Could you check a few things on this model? Use its own coordinates, in mm. Give positions to 0.01 mm unless a question says otherwise; leave off trailing zeros. Order: outer loops, then holes, each group sorted by start corner. A loop starts at its lowest first (then second) coordinate and runs counter-clockwise, first axis right, second up. Notation, with made-up numbers: M 56.25,66.25 L 110.25,66.25 A24 ccw 110.25,98.25 Z; hole C 52.5,12.25 d1. An arc over 180 degrees is marked long. Use a Markdown table: item, result. Add a question column.
Item 1: If I drill on L1, parallel to Y at x = 4.75, z = -1.5; L2, parallel to X at y = -14, z = 4.5; L3, parallel to Y at x = 6.5, z = -1.25, over which ranges is the centre line in solid material (lowest first)? Write a range as from..to.
Item 2: I'm going to push flat-ended pins straight in: pin 1 Ø0.6 at (x, y) = (1, -99) entering from +Z; pin 2 Ø2 at (y, z) = (-168, -12) entering from -X; pin 3 Ø1.5 at (x, y) = (4, -85.5) entering from +Z. Where does each tip first touch, or does it pass through?
Item 3: If we mould it in two halves opening along Z, with no side actions, what happens to faces 1 (the face through (4.056, -249.768, -3.294)), 2 (the face through (5, -271.216, -2)), 3 (the face through (4.056, -242.268, -3.294))? For each: released by +Z, released by -Z, zero draft, split by the parting line, or undercut.
Item 4: Suppose I cut it at B-B on x = 3.5. Write out the boundary of the cut face in (y, z).
Item 5: Suppose I cut it at A-A on y = -134.5. Write out the boundary of the cut face in (x, z), plus the area to 3 significant figures.
from build123d import *

# Parameters (mm, degrees)
CROQUIS1_W              = 25
CROQUIS1_H              = 300
SALIENTE_EXTRUIR1_DEPTH = 8
CORTAR_EXTRUIR1_DEPTH   = 301.454304751
CROQUIS3_R              = 2.5
CORTAR_EXTRUIR2_DEPTH   = 272.718032041


with BuildPart() as part:
    # Croquis1 → Saliente-Extruir1 (new body)
    with BuildSketch(Plane(origin=(0, 0, 0), x_dir=(0, 0, -1), z_dir=(1, 0, 0))):
        with Locations((1.949541284, -121.21559633)):
            Rectangle(CROQUIS1_W, CROQUIS1_H)
    extrude(amount=SALIENTE_EXTRUIR1_DEPTH)

    # Croquis2 → Cortar-Extruir1 (cut, through all)
    with BuildSketch(Plane(origin=(0, 28.78440367, 0), x_dir=(1, 0, 0), z_dir=(0, 1, 0))):
        Polygon((2, 8.451958984), (2, 7.451958984), (5, 7.451958984), (5, 14.449541284), (0, 14.449541284), (0, 8.451958984), align=None)
        Polygon((5, -10.550458716), (0, -10.550458716), (0, -4.552876416), (2, -4.552876416), (2, -3.552876416), (5, -3.552876416), align=None)
    extrude(amount=-CORTAR_EXTRUIR1_DEPTH, mode=Mode.SUBTRACT)

    # Croquis3 → Cortar-Extruir2 (cut, through all)
    with BuildSketch(Plane(origin=(8, 0, 0), x_dir=(0, 0, -1), z_dir=(1, 0, 0))):
        with Locations((1.949541284, -251.876037927)):
            Circle(CROQUIS3_R)
        with Locations((1.949541284, -244.376037927)):
            Circle(CROQUIS3_R)
    extrude(amount=-CORTAR_EXTRUIR2_DEPTH, mode=Mode.SUBTRACT)


solid = part.part
Findings below:
| question | item | result |
|---|---|---|
| 1 | L1 | y = -271.22..-254.34, -249.42..-246.84, -241.92..28.78 |
| 1 | L2 | x = 0..2, 5..8 |
| 1 | L3 | y = -271.22..-254.28, -249.48..-246.78, -241.98..28.78 |
| 2 | pin 1 | stops at z = 4.55 |
| 2 | pin 2 | stops at x = 5 |
| 2 | pin 3 | stops at z = 3.55 |
| 3 | face 1 | undercut |
| 3 | face 2 | zero draft |
| 3 | face 3 | undercut |
| 4 | outline | M -271.22,-7.45 L 28.78,-7.45 L 28.78,3.55 L -271.22,3.55 Z; hole C -251.88,-1.95 d5; hole C -244.38,-1.95 d5 |
| 5 | outline | M 0,-8.45 L 2,-8.45 L 2,-7.45 L 5,-7.45 L 5,-14.45 L 8,-14.45 L 8,10.55 L 5,10.55 L 5,3.55 L 2,3.55 L 2,4.55 L 0,4.55 Z |
| 5 | area | 134 mm^2 |
